The drawing under review shows one solid part. Ordinate dimensions are in mm from its lowest x, y, z. Round coordinates to 2 decimals unless told otherwise and drop trailing zeros. Loops run counter-clockwise (first coordinate to the right, second up) from the corner with the lowest first, then second, coordinate; pieces in that order, holes last. Notation, with made-up numbers: (8, 54.5) -> (54, 54.5) arc R34 ccw to (54, 90.5) -> close; hole circle Ø3 at (-25, 20.5). An arc over 180 degrees is marked (long way). Use a Markdown table: item, result. Add a question column.
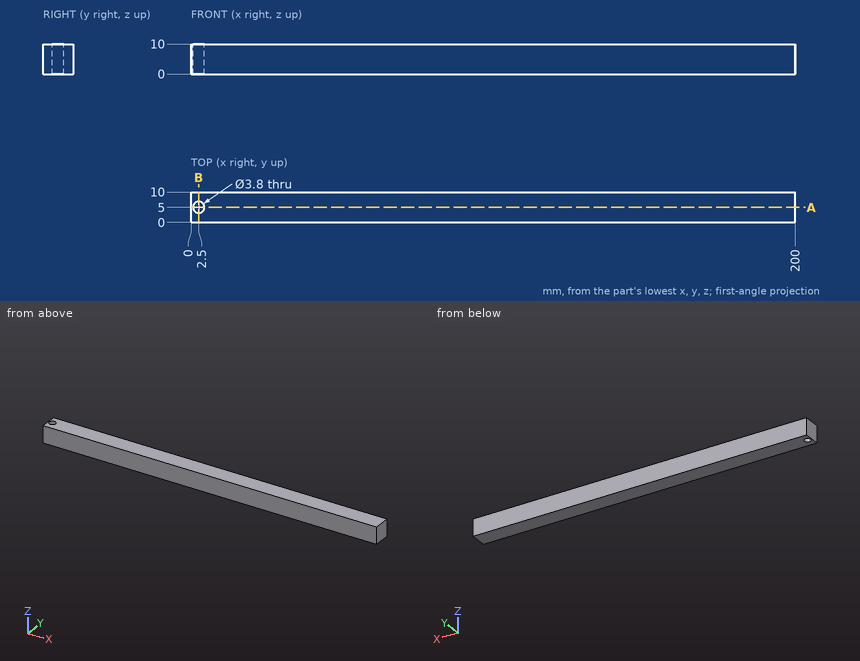
1. Consider section A-A on y = 5. State the section outline as (x, z) points, plus the area to 3 significant figures.
2. Insertion check: P1, Ø3.5, axis at x = 2.5, y = 5, coming from the -Z side. The pin has a flat end and moves straight along its axis. Give the tip position at first contact, or say it passes through.
3. To check wall thickness, follow probe 1 along Y at (x, z) = (2.5, 8); probe 2 along X at (y, z) = (4.5, 7); probe 3 along X at (y, z) = (5.25, 1.75). State the ranges of each line that lie inside material, in increasing order. Write a range as from..to.
4. Consider section B-B on x = 2.5. State the section outline as (y, z) points.
Verdict:
| question | item | result |
|---|---|---|
| 1 | outline | (0, 0) -> (0.6, 0) -> (0.6, 10) -> (0, 10) -> close; (4.4, 0) -> (200, 0) -> (200, 10) -> (4.4, 10) -> close |
| 1 | area | 1,960 mm² |
| 2 | P1 | passes through |
| 3 | probe 1 | y = 0..3.1, 6.9..10 |
| 3 | probe 2 | x = 0..0.67, 4.33..200 |
| 3 | probe 3 | x = 0..0.62, 4.38..200 |
| 4 | outline | (0, 0) -> (3.1, 0) -> (3.1, 10) -> (0, 10) -> close; (6.9, 0) -> (10, 0) -> (10, 10) -> (6.9, 10) -> close |
